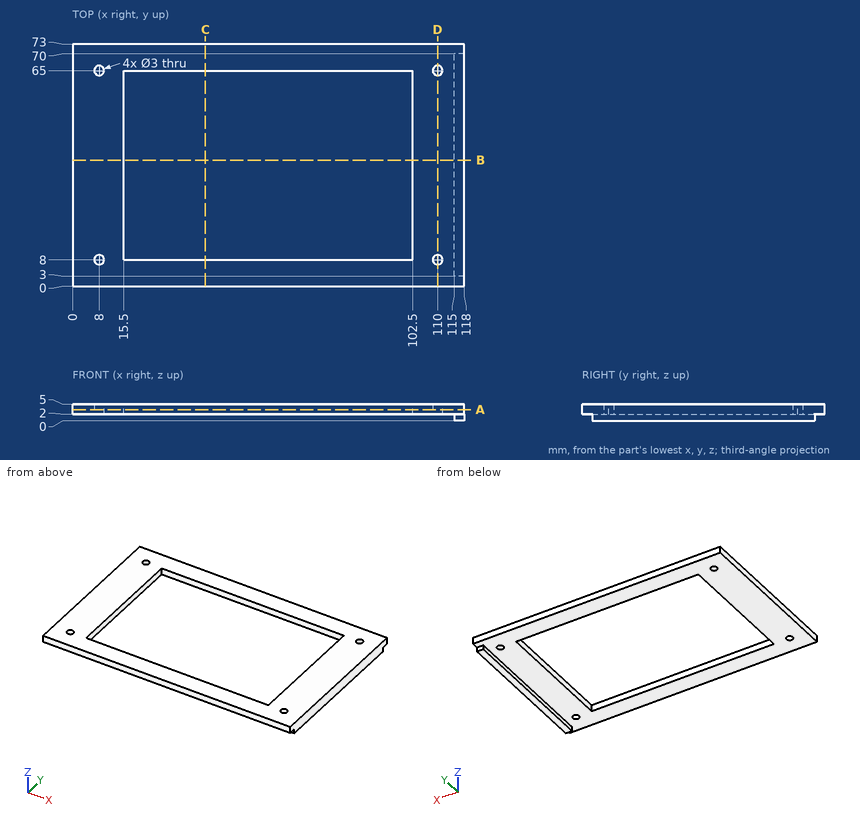
Could you check a few things on this drawing? It's one solid part, dimensions in mm from its lowest x, y, z. Give positions to 0.01 mm unless a question says otherwise; leave off trailing zeros. Order: outer loops, then holes, each group sorted by start corner. A loop starts at its lowest first (then second) coordinate and runs counter-clockwise, first axis right, second up. Notation, with made-up numbers: (22, 28) -> (47, 28) arc R27 ccw to (47, 50) -> close; hole circle Ø9 at (-20.5, -35). An arc over 180 degrees is marked (long way). Answer in a Markdown table with one row per item. Add a question column.
Item 1: Please list where these lines run through material, in increasing order: probe 1 along Y at (x, z) = (110, 3.95); probe 2 along X at (y, z) = (53.5, 2.55); probe 3 along Y at (x, z) = (81.5, 2.2).
Item 2: Imagine slicing it at D-D (x = 110). List the corners of the cut face in (y, z) for me.
Item 3: Imagine slicing it at A-A (z = 3.4). List the corners of the cut face in (x, y) for me.
Item 4: Imagine slicing it at B-B (y = 38). List the corners of the cut face in (x, z) for me, and give its area (3 significant figures).
Item 5: I'm going to push flat-ended pins straight in: P1, Ø4, axis at x = 8, y = 65, coming from the -Z side; P2, Ø2.5, axis at x = 110, y = 8, coming from the +Z side; P3, Ø0.6, axis at x = 116, z = 1.5, coming from the -Y side. Where does each tip first touch, or does it pass through?
Item 6: Imagine slicing it at C-C (x = 40). List the corners of the cut face in (y, z) for me, and give its area (3 significant figures).
Result:
| question | item | result |
|---|---|---|
| 1 | probe 1 | 0 to 6.5, 9.5 to 63.5, 66.5 to 73 |
| 1 | probe 2 | 0 to 15.5, 102.5 to 118 |
| 1 | probe 3 | 0 to 8, 65 to 73 |
| 2 | outline | (0, 2) -> (6.5, 2) -> (6.5, 5) -> (0, 5) -> close; (9.5, 2) -> (63.5, 2) -> (63.5, 5) -> (9.5, 5) -> close; (66.5, 2) -> (73, 2) -> (73, 5) -> (66.5, 5) -> close |
| 3 | outline | (0, 0) -> (118, 0) -> (118, 73) -> (0, 73) -> close; hole circle Ø3 at (8, 8); hole circle Ø3 at (8, 65); hole (15.5, 8) -> (102.5, 8) -> (102.5, 65) -> (15.5, 65) -> close; hole circle Ø3 at (110, 8); hole circle Ø3 at (110, 65) |
| 4 | outline | (0, 2) -> (15.5, 2) -> (15.5, 5) -> (0, 5) -> close; (102.5, 2) -> (115, 2) -> (115, 0) -> (118, 0) -> (118, 5) -> (102.5, 5) -> close |
| 4 | area | 99.0 mm2 |
| 5 | P1 | z = 2 |
| 5 | P2 | through |
| 5 | P3 | y = 3 |
| 6 | outline | (0, 2) -> (8, 2) -> (8, 5) -> (0, 5) -> close; (65, 2) -> (73, 2) -> (73, 5) -> (65, 5) -> close |
| 6 | area | 48.0 mm2 |
